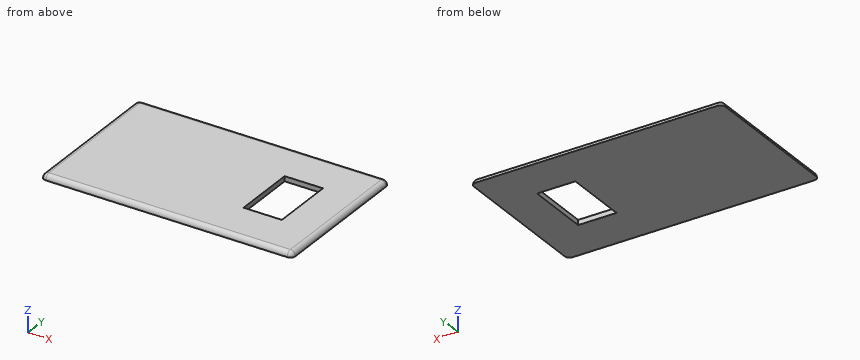
```python
from build123d import *

# Parameters (mm, degrees)
SKETCH1_W           = 100
SKETCH1_H           = 60
BOSS_EXTRUDE1_DEPTH = 2
FILLET1_R           = 2
SKETCH2_W           = 15.24
SKETCH2_H           = 25.4
CUT_EXTRUDE1_DEPTH  = 59.343808583


with BuildPart() as part:
    # Sketch1 → Boss-Extrude1 (new body)
    with BuildSketch(Plane.XY):
        Rectangle(SKETCH1_W, SKETCH1_H)
    extrude(amount=BOSS_EXTRUDE1_DEPTH)

    # Fillet1
    fillet1_edges = [part.edges().sort_by_distance(p)[0] for p in [
        (0, 30, 2),
        (-50, 0, 2),
        (0, -30, 2),
        (50, 0, 2),
        (-50, -30, 1),
        (-50, 30, 1),
        (50, 30, 1),
        (50, -30, 1),
    ]]
    fillet(fillet1_edges, radius=FILLET1_R - 0.0001)  # a hair under: the kernel refuses the full size

    # Sketch2 → Cut-Extrude1 (cut, through all)
    with BuildSketch(Plane.XY.offset(2)):
        with Locations((27.14, 0)):
            Rectangle(SKETCH2_W, SKETCH2_H)
    extrude(amount=-CUT_EXTRUDE1_DEPTH, mode=Mode.SUBTRACT)


solid = part.part
```
Can you work these out from the model? Positions are in its coordinate system, mm. Coordinates: 2 decimals unless noted, no trailing zeros. Loops run counter-clockwise (first coordinate to the right, second up) from the corner with the lowest first, then second, coordinate; pieces in that order, holes last. Notation, with made-up numbers: (38.5, 85) -> (67.5, 85) arc R24 ccw to (67.5, 106) -> close; hole circle Ø11 at (53.25, -36). An arc over 180 degrees is marked (long way). Answer as a JSON object with one key per item and string values.
1) For P1, Ø1, axis at x = 30.5, z = 1.5, coming from the -Y side; P2, Ø1, axis at x = 25.5, z = 1.5, coming from the +Y side, each with a flat end and sliding along its axis, tell me the tip position at first contact or that it passes through.
Results:
{"P1": "stops at y = -29.73", "P2": "stops at y = 29.73"}
2) Imagine slicing it at C-C (z = 0.35). Please give me the cut outline in (x, y).
Results:
{"outline": "(-49.97, -28) arc R1.97 ccw to (-48, -29.97) -> (48, -29.97) arc R1.97 ccw to (49.97, -28) -> (49.97, 28) arc R1.97 ccw to (48, 29.97) -> (-48, 29.97) arc R1.97 ccw to (-49.97, 28) -> close; hole (19.52, -12.7) -> (34.76, -12.7) -> (34.76, 12.7) -> (19.52, 12.7) -> close"}
3) If I drill on line 1 (X direction, y = -2.5, z = 0.3); line 2 (Y direction, x = 29, z = 0.2); line 3 (Y direction, x = 32, z = 1.75), over which ranges is the centre line in solid material (lowest first)?
Results:
{"line 1": "x = -49.98 to 19.52, 34.76 to 49.98", "line 2": "y = -29.99 to -12.7, 12.7 to 29.99", "line 3": "y = -28.97 to -12.7, 12.7 to 28.97"}
